from build123d import *

# Parameters (mm, degrees)
SKETCH1_W = 44.45
SKETCH1_H = 3.175
FILLET1_R = 0.254


with BuildPart() as part:
    # Sketch1 → Revolve1 (revolve)
    with BuildSketch(Plane(origin=(0, 0, 0), x_dir=(0, 0, -1), z_dir=(1, 0, 0))):
        with Locations((0, 1.5875)):
            Rectangle(SKETCH1_W, SKETCH1_H)
    revolve(axis=Axis((0, 0, 8.5598), (0, 0, 1)))

    # Sketch5 → Revolve3 (revolve)
    with BuildSketch(Plane(origin=(0, 0, 0), x_dir=(0, 0, -1), z_dir=(1, 0, 0))):
        Polygon((-22.225, 7.9375), (-34.925, 7.9375), (-34.925, 12.7), (-41.275, 12.7), (-41.275, 0), (-22.225, 0), align=None)
    revolve(axis=Axis((0, 0, 22.225), (0, 0, -1)))

    # Sketch11 → Cut-Revolve4 (revolve, cut)
    with BuildSketch(Plane(origin=(0, 0, 0), x_dir=(0, 0, -1), z_dir=(1, 0, 0))):
        Polygon((21.317857143, 3.175), (22.225, 2.751992339), (22.225, 3.175), align=None)
    revolve(axis=Axis((0, 0, 0), (0, 0, -1)), mode=Mode.SUBTRACT)

    # Fillet1
    fillet1_edges = [part.edges().sort_by_distance(p)[0] for p in [
        (0, -7.9375, 22.225),
        (0, -12.7, 34.925),
        (0, -12.7, 41.275),
    ]]
    fillet(fillet1_edges, radius=FILLET1_R)


solid = part.part
The model under review builds one solid part; all positions refer to its coordinate system, in mm. A direction names the side the tool comes from. Round coordinates to 2 decimals unless told otherwise and drop trailing zeros. Write each loop counter-clockwise with the first axis right and the second up, starting at its lowest first coordinate (ties: lowest second). Pieces come first, ordered by that corner, then holes. Notation, with made-up numbers: M -12.5,36.25 L 46.5,36.25 A27 cw 46.5,58.25 Z; hole C 70,24.25 d8. An arc over 180 degrees is marked long. Answer as CSV lines item,"result". Start each with the question number.
Q1. Wall thickness on line 1 along Z through (x, y) = (1, 7.5) (3 decimals); line 2 along Z through (x, y) = (6.25, -9.25) (3 decimals); line 3 along Y through (x, z) = (-0.25, -2): over which ranges is each line inside the solid? List them lowest first.
Q2. Clearance check with flat-ended pins moving along their axes: P1, Ø2, axis at y = -5, z = 24, coming from the +X side; P2, Ø1.5, axis at x = 8.5, y = -8.5, coming from the -Z side (3 decimals); P3, Ø4, axis at x = 4, y = 8.5, coming from the -Z side (3 decimals); P4, Ø4, axis at x = -9.5, z = 19.5, coming from the +Y side. State where each tip first meets the part, or that it passes through.
Q3. Consider section C-C, the plane z = 24. Give the boundary of the cut face in (x, y) (1 decimal).
Q4. Tool access review of faces 1 (the face through (-12.4, -2.75, 38.14)), 2 (the face through (-7.75, -1.72, 28.79)): name each direction out of +Z, -Z, +X, -X, +Y, -Y from which nothing blocks a thin tool from reaching the whole face with its end or side.
Q5. Consider section D-D, the plane z = 5. Give the boundary of the cut face in (x, y) (3 decimals).
Result set:
1,line 1,"z = 22.225 to 41.275"
1,line 2,"z = 34.925 to 41.275"
1,line 3,"y = -3.17 to 3.17"
2,P1,"stops at x = 6.86"
2,P2,"stops at z = 34.925"
2,P3,"stops at z = 22.225"
2,P4,"passes through"
3,outline,"C 0,0 d15.9"
4,face 1,"+Z, -Z"
4,face 2,"-Z"
5,outline,"C 0,0 d6.35"
